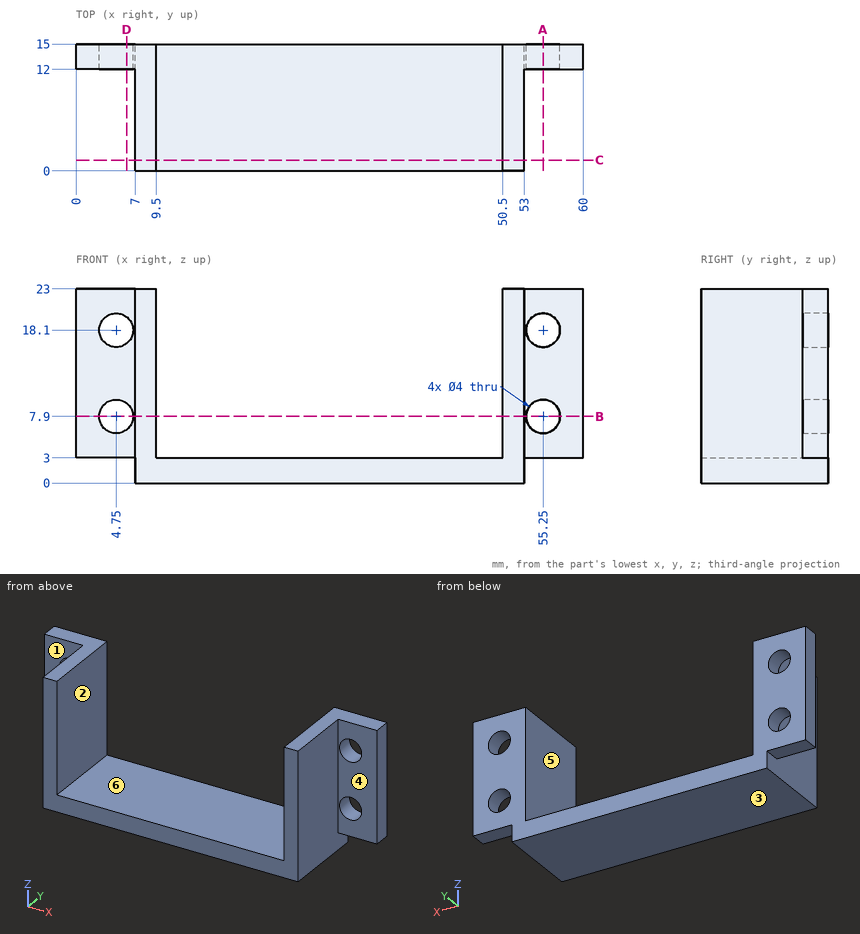
Geometry: see drawing. Coordinates: mm, zero at the bounding-box minimum. A direction names the side the tool comes from. Give positions to 0.01 mm unless a question says otherwise; leave off trailing zeros. Write each loop counter-clockwise with the first axis right and the second up, starting at its lowest first coordinate (ties: lowest second). Pieces come first, ordered by that corner, then holes. Notation, with made-up numbers: M 14.5,49.5 L 71.5,49.5 A29 cw 71.5,77.5 Z; hole C -16.75,67.5 d8. An arc over 180 degrees is marked long. Return JSON: item names as keys, results as strings. Group by question number.
1) Cut plane C-C, the plane y = 1.25. Output: boundary loops of the cut face in (x, z), then the cut area to 3 significant figures.
2) First-contact query: pin 1 Ø5.5 at (x, z) = (3, 17) entering from -Y; pin 2 Ø2.5 at (x, y) = (55.5, 13) entering from -Z; pin 3 Ø8 at (y, z) = (3.5, 12) entering from -X. Flat tips, straight axial feed; report the tip coordinate or a pass-through.
3) Cut plane D-D, the plane x = 6. Output: boundary loops of the cut face in (y, z).
4) Cut plane A-A, the plane x = 55.25. Output: boundary loops of the cut face in (y, z), then the cut area to 3 significant figures.
5) Draft query along X for the marked faces 4, 5 and 6. Return one class per face: released by +X, released by -X, zero draft, split by the parting line, or undercut.
6) Ray query, L1, parallel to X at y = 14.35, z = 7.9; L2, parallel to Z at x = 55.25, y = 12.7; L3, parallel to X at y = 8.5, z = 8.75. Return the intervals inside material, ascending.
7) Set-up query: the marked faces 1, 2 and 3. Return all of +Z, -Z, +X, -X, +Y, -Y with unobstructed straight access to the full face (end or side cutting, diameter ignored); none if empty.
8) Cut plane B-B, the plane z = 7.9. Output: boundary loops of the cut face in (x, y), then the cut area to 3 significant figures.
Data:
{
 "1": {"outline": "M 7,0 L 53,0 L 53,23 L 50.5,23 L 50.5,3 L 9.5,3 L 9.5,23 L 7,23 Z", "area": "238 mm²"},
 "2": {"pin 1": "stops at y = 12", "pin 2": "stops at z = 3", "pin 3": "stops at x = 7"},
 "3": {"outline": "M 12,3 L 15,3 L 15,6.34 L 12,6.34 Z; M 12,9.46 L 15,9.46 L 15,16.54 L 12,16.54 Z; M 12,19.66 L 15,19.66 L 15,23 L 12,23 Z"},
 "4": {"outline": "M 12,3 L 15,3 L 15,5.9 L 12,5.9 Z; M 12,9.9 L 15,9.9 L 15,16.1 L 12,16.1 Z; M 12,20.1 L 15,20.1 L 15,23 L 12,23 Z", "area": "36.0 mm²"},
 "5": {"face 4": "zero draft", "face 5": "undercut", "face 6": "undercut"},
 "6": {"L1": "x = 0 to 2.75, 6.75 to 9.5, 50.5 to 53.25, 57.25 to 60", "L2": "z = 3 to 5.9, 9.9 to 16.1, 20.1 to 23", "L3": "x = 7 to 9.5, 50.5 to 53"},
 "7": {"face 1": "+Z, -Z, -X, -Y", "face 2": "+Z, +Y, -Y", "face 3": "-Z, +X, -X, +Y, -Y"},
 "8": {"outline": "M 0,12 L 2.75,12 L 2.75,15 L 0,15 Z; M 6.75,12 L 7,12 L 7,0 L 9.5,0 L 9.5,15 L 6.75,15 Z; M 50.5,0 L 53,0 L 53,12 L 53.25,12 L 53.25,15 L 50.5,15 Z; M 57.25,12 L 60,12 L 60,15 L 57.25,15 Z", "area": "93.0 mm²"}
}
